from build123d import *

# Parameters (mm, degrees)
SKETCH1_R           = 1.5
BOSS_EXTRUDE1_DEPTH = 1.6
SKETCH2_R           = 1.5
CUT_EXTRUDE1_DEPTH  = 2.6
SKETCH3_R           = 2.5
BOSS_EXTRUDE2_DEPTH = 14.1
SKETCH4_R           = 2.5
BOSS_EXTRUDE3_DEPTH = 21.25


with BuildPart() as part:
    # Sketch1 → Boss-Extrude1 (new body)
    with BuildSketch(Plane.XY):
        with BuildLine():
            Line((0, 0), (0, 68.543560763))
            Line((0, 68.543560763), (10, 68.543560763))
            Line((10, 68.543560763), (10, 0))
            ThreePointArc((10, 0), (5, -23.956439237), (0, 0))
        make_face()
        with Locations((5, -11.456439237)):
            Circle(SKETCH1_R, mode=Mode.SUBTRACT)
    extrude(amount=BOSS_EXTRUDE1_DEPTH)

    # Sketch2 → Cut-Extrude1 (cut, through all)
    with BuildSketch(Plane.XY.offset(1.6)):
        with Locations((5, 63.543560763)):
            Circle(SKETCH2_R)
    extrude(amount=-CUT_EXTRUDE1_DEPTH, mode=Mode.SUBTRACT)

    # Sketch3 → Boss-Extrude2 (add)
    with BuildSketch(Plane.XY.offset(1.6)):
        with Locations((5, 36.043560763)):
            Circle(SKETCH3_R)
    extrude(amount=BOSS_EXTRUDE2_DEPTH)

    # Sketch4 → Boss-Extrude3 (add)
    with BuildSketch(Plane(origin=(0, 0, 0), x_dir=(-1, 0, 0), z_dir=(0, 0, -1))):
        with Locations((-5, 36.043560763)):
            Circle(SKETCH4_R)
    extrude(amount=BOSS_EXTRUDE3_DEPTH)


solid = part.part
The listing builds one solid part. Answer for the finished solid, in the listing's coordinates (mm). A direction names the side the tool comes from. Coordinates: 2 decimals unless noted, no trailing zeros. Loops run counter-clockwise (first coordinate to the right, second up) from the corner with the lowest first, then second, coordinate; pieces in that order, holes last. Notation, with made-up numbers: (75, 14) -> (100, 14) arc R18 ccw to (100, 46) -> close; hole circle Ø9 at (45.25, -40). An arc over 180 degrees is marked (long way). Write item = value, one per line. Start each with the question number.
1) A cutting plane is placed at D-D (z = -4.5). Give the vertices of the cut face in (x, y), then the cut area to 3 significant figures.
2) The mould has two halves that part along X. Classify faces 1 (the face through (5.478, -23.947, 0.789)), 2 (the face through (5.806, 64.808, 0.811)), 3 (the face through (5, 36, 15.7)): released by +X, released by -X, zero draft, split by the parting line, or undercut.
3) Given pin 1 Ø1.3 at (y, z) = (17.5, 1) entering from +X; pin 2 Ø1.5 at (x, y) = (7.5, 32) entering from +Z; pin 3 Ø10 at (y, z) = (32, 6.5) entering from -X; pin 4 Ø2 at (x, z) = (0.5, -5.5) entering from +Y, each flat-ended and moving along its own axis, determine where each tip first touches the part or whether it passes through.
4) A tool of negligible diameter and unlimited length cuts with its end or side. For faces 4 (the face through (4.458, 33.603, 8.551)), 5 (the face through (5, 36, -21.25)), 6 (the face through (5.542, 33.603, -10.476)), 7 (the face through (10, 35, 1)), 8 (the face through (0, 34, 1)), from which of +Z, -Z, +X, -X, +Y, -Y can it reach the whole face along a straight path? Write none if from no direction.
5) Straight lines are drawn through the part: line 1 (Y direction, x = 5, z = 1.3); line 2 (Z direction, x = 5.5, y = 29); line 3 (X direction, y = 38, z = 8). For each, find the intervals that lie inside material, in ascending order. Write a range as from..to.
6) A cutting plane is placed at A-A (x = 5). Give the vertices of the cut face in (y, z).
7) A cutting plane is placed at C-C (x = 15.5). Give the vertices of the cut face in (y, z).
8) A cutting plane is placed at B-B (y = 9). Give the vertices of the cut face in (x, z).
Responses:
q1.outline = circle Ø5 at (5, 36.04)
q1.area = 19.6 mm²
q2.face_1 = split by the parting line
q2.face_2 = undercut
q2.face_3 = zero draft
q3.pin_1 = 10
q3.pin_2 = 1.6
q3.pin_3 = 0
q3.pin_4 = through
q4.face_4 = +Z
q4.face_5 = -Z, +X, -X, +Y, -Y
q4.face_6 = -Z
q4.face_7 = +Z, -Z, +X, +Y
q4.face_8 = +Z, -Z, -X, +Y
q5.line_1 = -23.96..-12.96, -9.96..62.04, 65.04..68.54
q5.line_2 = 0..1.6
q5.line_3 = 3.44..6.56
q6.outline = (-23.96, 0) -> (-12.96, 0) -> (-12.96, 1.6) -> (-23.96, 1.6) -> close; (-9.96, 0) -> (33.54, 0) -> (33.54, -21.25) -> (38.54, -21.25) -> (38.54, 0) -> (62.04, 0) -> (62.04, 1.6) -> (38.54, 1.6) -> (38.54, 15.7) -> (33.54, 15.7) -> (33.54, 1.6) -> (-9.96, 1.6) -> close; (65.04, 0) -> (68.54, 0) -> (68.54, 1.6) -> (65.04, 1.6) -> close
q7.outline = (-18.24, 0) -> (-4.67, 0) -> (-4.67, 1.6) -> (-18.24, 1.6) -> close
q8.outline = (0, 0) -> (10, 0) -> (10, 1.6) -> (0, 1.6) -> close
